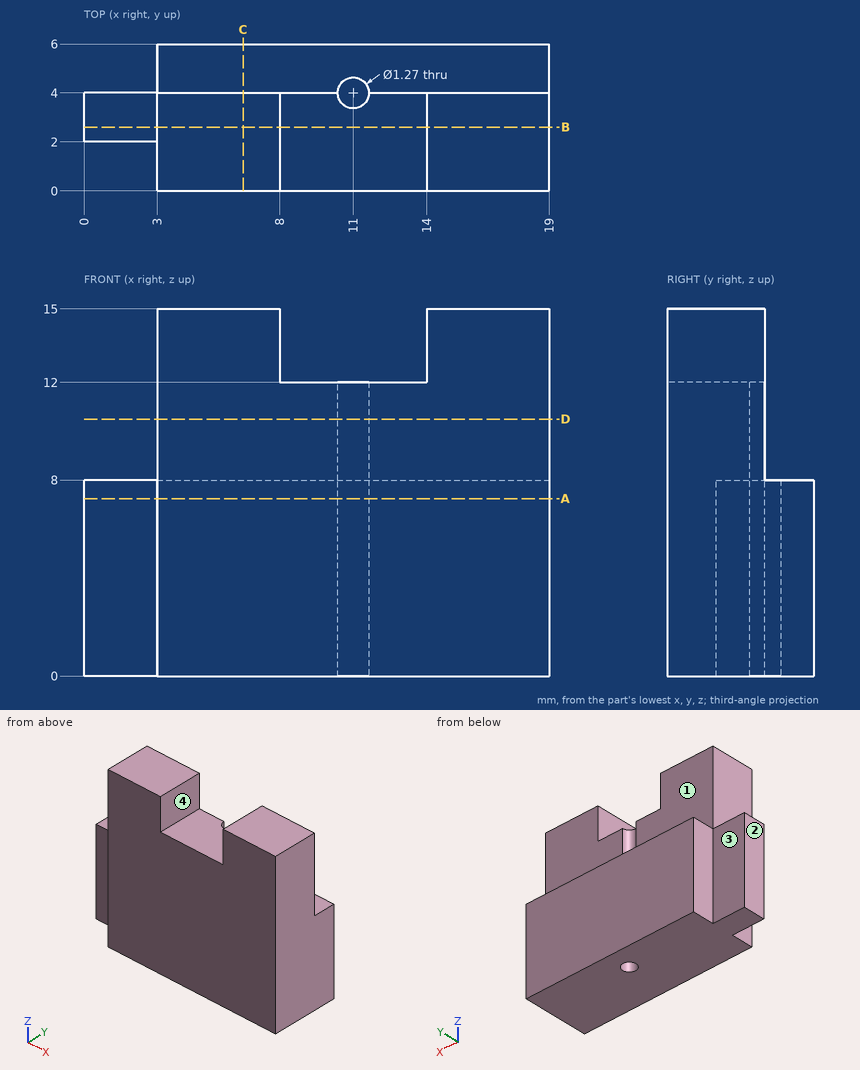
Geometry check sheet. Reference: drawing and pictorial views, mm from the part's lowest x, y, z. A direction names the side the tool comes from. Round coordinates to 2 decimals unless told otherwise and drop trailing zeros. Write each loop counter-clockwise with the first axis right and the second up, starting at its lowest first coordinate (ties: lowest second). Pieces come first, ordered by that corner, then holes.
1. Gauge pin test, flat ends, axial feed: P1, Ø2, axis at x = 16.5, z = 11, coming from the +Y side; P2, Ø2.5, axis at x = 1, z = 5.5, coming from the -Y side; P3, Ø0.9, axis at y = 2.5, z = 13, coming from the -X side; P4, Ø1, axis at x = 11, y = 4, coming from the +Z side. Record the tip position at first contact, or that the pin passes through.
2. Section check B-B on y = 2.6. Enter the section's corners in (x, z).
3. Section check D-D on z = 10.5. Enter the section's corners in (x, y) (3 decimals).
4. Access from +Z, -Z, +X, -X, +Y, -Y to the whole of each face (thin tool, end or side, straight path). Record for the marked faces 1, 2, 3 and 4.
5. Section check A-A on z = 7.25. Enter the section's corners in (x, y) (3 decimals), plus the area to 3 significant figures.
6. Scan lines: L1, parallel to X at y = 2.8, z = 13.75; L2, parallel to Z at x = 12.75, y = 1.75; L3, parallel to Z at x = 1, y = 3.3. Record each from-to range of solid material in increasing order.
7. Section check C-C on x = 6.5. Enter the section's corners in (y, z), plus the area to 3 significant figures.
Answer:
1. P1: stops at y = 4
1. P2: stops at y = 2
1. P3: stops at x = 3
1. P4: passes through
2. outline: (0, 0) - (19, 0) - (19, 15) - (14, 15) - (14, 12) - (8, 12) - (8, 15) - (3, 15) - (3, 8) - (0, 8) - close
3. outline: (3, 0) - (19, 0) - (19, 4) - (11.635, 4) arc R0.635 cw to (10.365, 4) - (3, 4) - close
4. face 1: +Z, +X, -X, +Y
4. face 2: +Z, -Z, -X, +Y, -Y
4. face 3: +Z, -Z, -X, +Y
4. face 4: +Z, +Y, -Y
5. outline: (0, 2) - (3, 2) - (3, 0) - (19, 0) - (19, 6) - (3, 6) - (3, 4) - (0, 4) - close; hole circle Ø1.27 at (11, 4)
5. area: 101 mm2
6. L1: x = 3 to 8, 14 to 19
6. L2: z = 0 to 12
6. L3: z = 0 to 8
7. outline: (0, 0) - (6, 0) - (6, 8) - (4, 8) - (4, 15) - (0, 15) - close
7. area: 76.0 mm2
